Autodesk Inventor part; units mm, degrees
ref_plane "YZ Plane" through (0, 0, 0) normal (1, 0, 0) x (0, 1, 0)
ref_plane "XZ Plane" through (0, 0, 0) normal (0, 1, 0) x (-1, 0, 0)
ref_plane "XY Plane" through (0, 0, 0) normal (0, 0, 1) x (1, 0, 0)
sketch "スケッチ1" plane through (0, 0, 0) normal (0, 0, 1) x (1, 0, 0)
  line L0 (2.75, 1.5877) -> (2.75, -1.5877)
  line L1 (2.75, -1.5877) -> (0, -3.1754)
  line L2 (0, -3.1754) -> (-2.75, -1.5877)
  line L3 (-2.75, -1.5877) -> (-2.75, 1.5877)
  line L4 (-2.75, 1.5877) -> (0, 3.1754)
  line L5 (0, 3.1754) -> (2.75, 1.5877)
  point P0 (0, 0)
  point P1 (0, 0)
  dimension "d0" = 5.5
extrude "押し出し1" add sketch "スケッチ1" along normal blind 29
sketch "スケッチ2" plane through (0, 0, 29) normal (0, 0, 1) x (1, 0, 0)
  point P0 (0, 0)
  point P1 (0, 0)
hole "穴1" at (0, 0, 29) direction (0, 0, -1) diameter 2.459 depth 6
mirror "ミラー1" about plane through (0, 0, 0) normal (0, 0, -1) of "押し出し1", "穴1"
properties part number "ASU-340" material "ステンレス鋼 AISI 304"
Work out the finished part from the listing and answer in its coordinate system (mm). A direction names the side the tool comes from. Coordinates: 2 decimals unless noted, no trailing zeros. Order: outer loops, then holes, each group sorted by start corner. A loop starts at its lowest first (then second) coordinate and runs counter-clockwise, first axis right, second up. Notation, with made-up numbers: (-19, 24) - (-7, 24) arc R31 ccw to (-7, 49) - close; hole circle Ø10 at (89.5, 9.5). An arc over 180 degrees is marked (long way). Put each result on its own line as item: value. Start each with the question number.
1) Find section D-D (y = -2.25). Give the vertices of the cut face in (x, z).
2) Flat-ended cylindrical pins translate along their axes: pin 1 (1.2 mm diameter, centred on x = -0.5, y = 0, fed in from +Z); pin 2 (0.7 mm diameter, centred on x = 0, y = -0.5, fed in from -Z). Find the tip coordinate at first contact, or state that the pin passes through.
3) Find section C-C (x = 0.7). Give the vertices of the cut face in (y, z), plus the area to 3 significant figures.
4) Find the intervals of material crossed by line 1 (Y direction, x = 0, z = 27.1); line 2 (Z direction, x = 0.65, y = 0); line 3 (X direction, y = 0, z = -26.4), in increasing order. Write a range as from..to.
5) For faces 4 (the flat face through (0, 0, -23)), 5 (the flat face through (0, 0, 23)), 6 (the flat face through (-2.75, 0, 0)), determine the directions among +Z, -Z, +X, -X, +Y, -Y from which every point of the face is accessible in a straight line to the end or side of a thin tool.
6) For a pull along Y with two mould halves and no side action, classify faces 1 (the flat face through (0, -1.4, 29)), 2 (the cylindrical face through (-0.748, 0.976, -25.958)), 3 (the flat face through (1.394, 2.37, 0.406)) as released by +Y, released by -Y, zero draft, split by the parting line, or undercut.
7) Find section B-B (y = 0). Give the vertices of the cut face in (x, z).
8) Find section A-A (z = -15). Give the vertices of the cut face in (x, y).
Results list:
1. outline: (-1.6, -29) - (1.6, -29) - (1.6, 29) - (-1.6, 29) - close
2. pin 1: stops at z = 23
2. pin 2: stops at z = -23
3. outline: (-2.77, -29) - (-1.01, -29) - (-1.01, -23) - (1.01, -23) - (1.01, -29) - (2.77, -29) - (2.77, 29) - (1.01, 29) - (1.01, 23) - (-1.01, 23) - (-1.01, 29) - (-2.77, 29) - close
3. area: 297 mm^2
4. line 1: y = -3.18..-1.23, 1.23..3.18
4. line 2: z = -23..23
4. line 3: x = -2.75..-1.23, 1.23..2.75
5. face 4: -Z
5. face 5: +Z
5. face 6: +Z, -Z, -X, +Y, -Y
6. face 1: zero draft
6. face 2: undercut
6. face 3: released by +Y
7. outline: (-2.75, -29) - (-1.23, -29) - (-1.23, -23) - (1.23, -23) - (1.23, -29) - (2.75, -29) - (2.75, 29) - (1.23, 29) - (1.23, 23) - (-1.23, 23) - (-1.23, 29) - (-2.75, 29) - close
8. outline: (-2.75, -1.59) - (0, -3.18) - (2.75, -1.59) - (2.75, 1.59) - (0, 3.18) - (-2.75, 1.59) - close
